Job drawing, mm, ordinate dimensions from the low corner. One solid piece. A direction names the side the tool comes from. Round coordinates to 2 decimals unless told otherwise and drop trailing zeros. Loops run counter-clockwise (first coordinate to the right, second up) from the corner with the lowest first, then second, coordinate; pieces in that order, holes last.
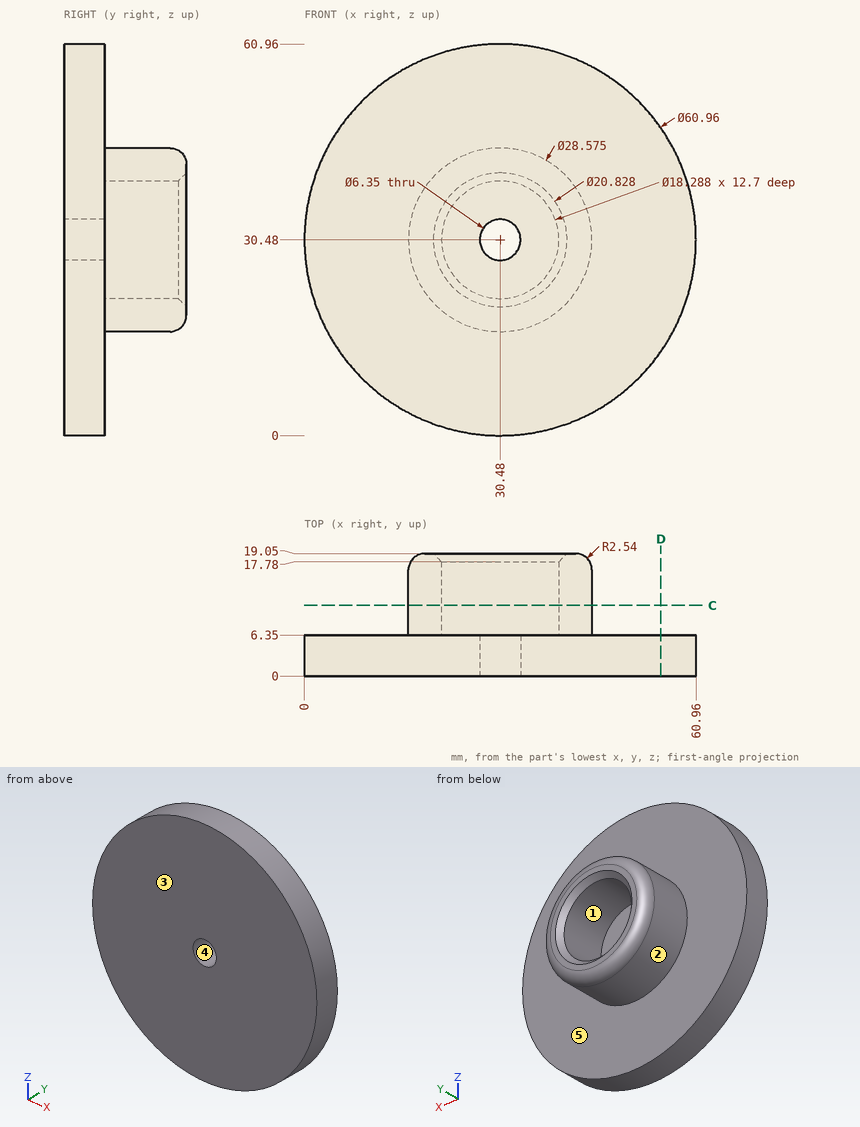
(1) Pull direction X, two halves, no side cores. Call the marked faces 1, 2 and 3: +X half, -X half, draft (parallel to the pull), parting line (faces both ways), or undercut.
Responses:
face 1: undercut
face 2: parting line
face 3: draft
(2) Pin check, flat tips, straight feed: P1, Ø2, axis at x = 31.5, y = 4, coming from the -Z side; P2, Ø9, axis at x = 33.5, z = 34.5, coming from the +Y side; P3, Ø1.5, axis at x = 12, z = 45.5, coming from the +Y side; P4, Ø4, axis at x = 30.48, z = 30.48, coming from the +Y side. Stop position of each tip, or through.
Responses:
P1: stops at z = 0
P2: stops at y = 18.16
P3: stops at y = 6.35
P4: passes through
(3) Probe line 1 (Z direction, x = 30.48, y = 9.5); line 2 (Y direction, x = 46, z = 41). List the from-to ranges inside material, lowest first.
Responses:
line 1: z = 16.19 to 21.34, 39.62 to 44.77
line 2: y = 0 to 6.35
(4) Slice it at C-C on y = 11. List the corners of the cut face in (x, z) (1 decimal).
Responses:
outline: circle Ø28.6 at (30.5, 30.5); hole circle Ø18.3 at (30.5, 30.5)
(5) Slice it at D-D on x = 55.5. List the corners of the cut face in (y, z).
Responses:
outline: (0, 13.07) - (6.35, 13.07) - (6.35, 47.89) - (0, 47.89) - close
(6) Which spindle directions (+Z, -Z, +X, -X, +Y, -Y) get a long thin tool onto all of the face, cutting with end or side? Do the marked faces 4 and 5. Say none if no direction does.
Responses:
face 4: +Y, -Y
face 5: +Y
